Verification items for the finished model (mm, model axes). A direction names the side the tool comes from. Round coordinates to 2 decimals unless told otherwise and drop trailing zeros. Order: outer loops, then holes, each group sorted by start corner. A loop starts at its lowest first (then second) coordinate and runs counter-clockwise, first axis right, second up. Notation, with made-up numbers: M 6.25,53.5 L 47.25,53.5 A14 ccw 47.25,78.5 Z; hole C 52.25,17 d4. An arc over 180 degrees is marked long. Write item = value, one per line. Start each with the question number.
from build123d import *

# Parameters (mm, degrees)
SKETCH1_W           = 95.25
SKETCH1_H           = 95.25
BOSS_EXTRUDE1_DEPTH = 17.78
SKETCH2_W           = 86.36
SKETCH2_H           = 8.89
CUT_EXTRUDE1_DEPTH  = 108.966807515
SKETCH3_R           = 12.7
CUT_EXTRUDE2_DEPTH  = 70.659239516
SKETCH4_R           = 3.175
CUT_EXTRUDE3_DEPTH  = 108.966807515


with BuildPart() as part:
    # Sketch1 → Boss-Extrude1 (new body)
    with BuildSketch(Plane.XY):
        Rectangle(SKETCH1_W, SKETCH1_H)
    extrude(amount=-BOSS_EXTRUDE1_DEPTH)

    # Sketch2 → Cut-Extrude1 (cut, through all)
    with BuildSketch(Plane(origin=(0, 47.625, 0), x_dir=(1, 0, 0), z_dir=(0, 1, 0))):
        with Locations((0, 8.89)):
            Rectangle(SKETCH2_W, SKETCH2_H)
    extrude(amount=-CUT_EXTRUDE1_DEPTH, mode=Mode.SUBTRACT)

    # Sketch3 → Cut-Extrude2 (cut, through all)
    with BuildSketch(Plane.XY):
        with Locations((19.05, 0)):
            Circle(SKETCH3_R)
        with Locations((-19.05, 0)):
            Circle(SKETCH3_R)
    extrude(amount=-CUT_EXTRUDE2_DEPTH, mode=Mode.SUBTRACT)

    # Sketch4 → Cut-Extrude3 (cut, through all)
    with BuildSketch(Plane(origin=(47.625, 0, 0), x_dir=(0, 0, -1), z_dir=(1, 0, 0))):
        with Locations((8.89, 10.16)):
            Circle(SKETCH4_R)
        with Locations((8.89, -10.16)):
            Circle(SKETCH4_R)
        with Locations((8.89, -27.94)):
            Circle(SKETCH4_R)
        with Locations((8.89, 27.94)):
            Circle(SKETCH4_R)
    extrude(amount=-CUT_EXTRUDE3_DEPTH, mode=Mode.SUBTRACT)


solid = part.part
1) Cross-section at C-C, the plane y = 10.16. Give the number of separate pieces and of enclosed holes in the cut face, then the cut area to 3 significant figures.
2) Scan lines: probe 1 along Y at (x, z) = (19.05, -15.45) (3 decimals); probe 2 along Y at (x, z) = (44.8, -8.89) (3 decimals); probe 3 along Z at (x, y) = (39, -20) (3 decimals). Record each from-to range of solid material in increasing order.
3) Cross-section at D-D, the plane z = -15.5. Enter the section's corners in (x, y) (3 decimals).
4) Release check for a two-part mould opening along Z. For faces 3 (the flat face through (-1, 1, 0)), 4 (the cylindrical face through (-6.936, 3.815, -2.191)), 5 (the cylindrical face through (-45.371, -30.757, -10.355)) record: pulls with the +Z half, pulls with the -Z half, needs draft (parallel to the pull), parting line crosses it, or undercut.
5) Access from +Z, -Z, +X, -X, +Y, -Y to the whole of each face (thin tool, end or side, straight path). Record for faces 1 (the flat face through (-1, 1, -13.335)), 2 (the cylindrical face through (31.164, 3.815, -2.191)).
6) Cross-section at B-B, the plane x = 8. Enter the section's corners in (y, z) (3 decimals), then the cut area to 3 significant figures.
7) Cross-section at A-A, the plane y = -27.94. Enter the section's corners in (x, z) (3 decimals).
Geometry results:
q1.separate_pieces = 6
q1.enclosed_holes = 0
q1.area = 598 mm^2
q2.probe_1 = -47.625 to -12.7, 12.7 to 47.625
q2.probe_2 = -47.625 to -31.115, -24.765 to -13.335, -6.985 to 6.985, 13.335 to 24.765, 31.115 to 47.625
q2.probe_3 = -17.78 to -13.335, -4.445 to 0
q3.outline = M -47.625,-47.625 L 47.625,-47.625 L 47.625,47.625 L -47.625,47.625 Z; hole C -19.05,0 d25.4; hole C 19.05,0 d25.4
q4.face_3 = pulls with the +Z half
q4.face_4 = needs draft
q4.face_5 = undercut
q5.face_1 = +Y, -Y
q5.face_2 = +Z, -Z
q6.outline = M -47.625,-17.78 L -6.26,-17.78 L -6.26,-13.335 L -47.625,-13.335 Z; M -47.625,-4.445 L -6.26,-4.445 L -6.26,0 L -47.625,0 Z; M 6.26,-17.78 L 47.625,-17.78 L 47.625,-13.335 L 6.26,-13.335 Z; M 6.26,-4.445 L 47.625,-4.445 L 47.625,0 L 6.26,0 Z
q6.area = 735 mm^2
q7.outline = M -47.625,-17.78 L 47.625,-17.78 L 47.625,-12.065 L 43.18,-12.065 L 43.18,-13.335 L -43.18,-13.335 L -43.18,-12.065 L -47.625,-12.065 Z; M -47.625,-5.715 L -43.18,-5.715 L -43.18,-4.445 L 43.18,-4.445 L 43.18,-5.715 L 47.625,-5.715 L 47.625,0 L -47.625,0 Z
